from build123d import *

# Parameters (mm, degrees)
SKETCH1_W           = 166
SKETCH1_H           = 96
BOSS_EXTRUDE1_DEPTH = 18
SKETCH2_W           = 150
SKETCH2_H           = 80
CUT_EXTRUDE1_DEPTH  = 15
CUT_EXTRUDE5_DEPTH  = 10
FILLET1_R           = 4
FILLET2_R           = 4
FILLET5_R           = 1
CHAMFER1_SIZE       = 0.5


with BuildPart() as part:
    # Sketch1 → Boss-Extrude1 (new body)
    with BuildSketch(Plane(origin=(0, 0, 0), x_dir=(1, 0, 0), z_dir=(0, 1, 0))):
        with Locations((18.075570249, -18.706715624)):
            Rectangle(SKETCH1_W, SKETCH1_H)
    extrude(amount=BOSS_EXTRUDE1_DEPTH)

    # Sketch2 → Cut-Extrude1 (cut)
    with BuildSketch(Plane(origin=(0, 18, 0), x_dir=(1, 0, 0), z_dir=(0, 1, 0))):
        with Locations((18.075570249, -18.706715624)):
            Rectangle(SKETCH2_W, SKETCH2_H)
    extrude(amount=-CUT_EXTRUDE1_DEPTH, mode=Mode.SUBTRACT)

    # Sketch9 → Cut-Extrude5 (cut)
    with BuildSketch(Plane(origin=(0, 18, 0), x_dir=(1, 0, 0), z_dir=(0, 1, 0))):
        Polygon((-62.174429751, 26.543284376), (98.325570249, 26.543284376), (98.325570249, -58.706715624), (95.325570249, -58.706715624), (95.325570249, 23.543284376), (-59.174429751, 23.543284376), (-59.174429751, -58.706715624), (-62.174429751, -58.706715624), align=None)
    extrude(amount=-CUT_EXTRUDE5_DEPTH, mode=Mode.SUBTRACT)

    # Fillet1
    fillet1_edges = [part.edges().sort_by_distance(p)[0] for p in [
        (-64.924429751, 9, -29.293284376),
        (101.075570249, 9, -29.293284376),
        (101.075570249, 9, 66.706715624),
        (-64.924429751, 9, 66.706715624),
    ]]
    fillet(fillet1_edges, radius=FILLET1_R)

    # Fillet2
    fillet2_edges = [part.edges().sort_by_distance(p)[0] for p in [
        (-56.924429751, 10.5, 58.706715624),
        (-56.924429751, 10.5, -21.293284376),
        (93.075570249, 10.5, -21.293284376),
        (93.075570249, 10.5, 58.706715624),
    ]]
    fillet(fillet2_edges, radius=FILLET2_R)

    # Fillet5
    fillet5_edges = [part.edges().sort_by_distance(p)[0] for p in [
        (-64.924429751, 18, 18.706715624),
        (18.075570249, 18, -29.293284376),
        (18.075570249, 18, 66.706715624),
        (101.075570249, 18, 18.706715624),
        (-63.752856875, 18, 65.535142749),
        (99.903997374, 18, 65.535142749),
        (99.903997374, 18, -28.1217115),
        (-63.752856875, 18, -28.1217115),
        (93.075570249, 18, 18.706715624),
        (18.075570249, 18, 58.706715624),
        (18.075570249, 18, -21.293284376),
        (-56.924429751, 18, 18.706715624),
        (91.903997374, 18, 57.535142749),
        (91.903997374, 18, -20.1217115),
        (-55.752856875, 18, -20.1217115),
        (-55.752856875, 18, 57.535142749),
    ]]
    fillet(fillet5_edges, radius=FILLET5_R)

    # Chamfer1
    chamfer1_edges = [part.edges().sort_by_distance(p)[0] for p in [
        (-62.174429751, 18, 16.081715624),
        (-60.674429751, 18, 58.706715624),
        (-59.174429751, 18, 17.581715624),
        (18.075570249, 18, -23.543284376),
        (95.325570249, 18, 17.581715624),
        (96.825570249, 18, 58.706715624),
        (98.325570249, 18, 16.081715624),
        (18.075570249, 18, -26.543284376),
    ]]
    chamfer(chamfer1_edges, length=CHAMFER1_SIZE)


solid = part.part
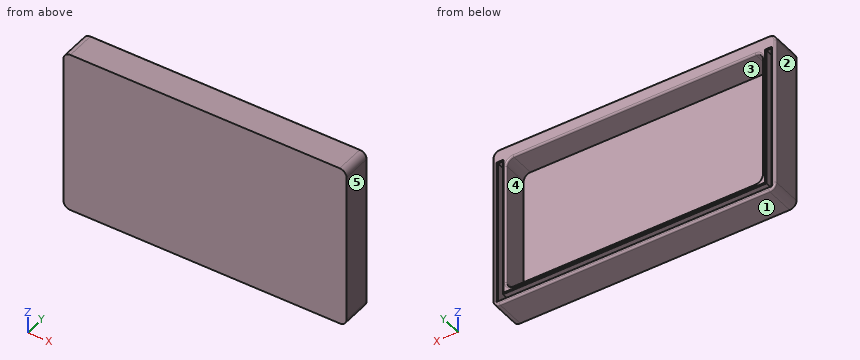
Read the model definition and answer for the solid it produces. Units are mm, in the model's axes. Face numbers are marked on the shaded views. A direction names the side the tool comes from. Coordinates: 2 decimals unless noted, no trailing zeros. Order: outer loops, then holes, each group sorted by start corner. A loop starts at its lowest first (then second) coordinate and runs counter-clockwise, first axis right, second up. Notation, with made-up numbers: (54.5, -11) -> (69.5, -11) arc R14 cw to (69.5, 0) -> close; hole circle Ø4 at (35, 47). An arc over 180 degrees is marked (long way). Answer as a JSON object with one key per item and string values.
1) A cutting plane is placed at D-D, the plane z = 49. Determine the outline of the cut face in (x, y).
Model answer:
{"outline": "(-64.92, 0) -> (101.08, 0) -> (101.08, 17) arc R1 ccw to (100.08, 18) -> (98.83, 18) -> (98.33, 17.5) -> (98.33, 8) -> (95.33, 8) -> (95.33, 17.5) -> (94.83, 18) -> (94.08, 18) arc R1 ccw to (93.08, 17) -> (93.08, 3) -> (-56.92, 3) -> (-56.92, 17) arc R1 ccw to (-57.92, 18) -> (-58.67, 18) -> (-59.17, 17.5) -> (-59.17, 8) -> (-62.17, 8) -> (-62.17, 17.5) -> (-62.67, 18) -> (-63.92, 18) arc R1 ccw to (-64.92, 17) -> close"}
2) The mould has two halves that part along Z. Classify the marked faces 1, 2 and 3: released by +Z, released by -Z, zero draft, split by the parting line, or undercut.
Model answer:
{"face 1": "released by -Z", "face 2": "zero draft", "face 3": "undercut"}
3) A tool of negligible diameter and unlimited length cuts with its end or side. For the marked faces 4 and 5, from which of +Z, -Z, +X, -X, +Y, -Y can it reach the whole face along a straight path? Write none if from no direction.
Model answer:
{"face 4": "+Y", "face 5": "+Z, -Z, +X, +Y, -Y"}
4) A cutting plane is placed at C-C, the plane y = 14.5. Determine the outline of the cut face in (x, z).
Model answer:
{"outline": "(-64.92, -25.29) arc R4 ccw to (-60.92, -29.29) -> (97.08, -29.29) arc R4 ccw to (101.08, -25.29) -> (101.08, 62.71) arc R4 ccw to (97.08, 66.71) -> (-60.92, 66.71) arc R4 ccw to (-64.92, 62.71) -> close; hole (-62.17, -26.54) -> (98.33, -26.54) -> (98.33, 58.71) -> (95.33, 58.71) -> (95.33, -23.54) -> (-59.17, -23.54) -> (-59.17, 58.71) -> (-62.17, 58.71) -> close; hole (-56.92, -17.29) arc R4 ccw to (-52.92, -21.29) -> (89.08, -21.29) arc R4 ccw to (93.08, -17.29) -> (93.08, 54.71) arc R4 ccw to (89.08, 58.71) -> (-52.92, 58.71) arc R4 ccw to (-56.92, 54.71) -> close"}
5) A cutting plane is placed at A-A, the plane y = 5.75. Determine the outline of the cut face in (x, z).
Model answer:
{"outline": "(-64.92, -25.29) arc R4 ccw to (-60.92, -29.29) -> (97.08, -29.29) arc R4 ccw to (101.08, -25.29) -> (101.08, 62.71) arc R4 ccw to (97.08, 66.71) -> (-60.92, 66.71) arc R4 ccw to (-64.92, 62.71) -> close; hole (-56.92, -17.29) arc R4 ccw to (-52.92, -21.29) -> (89.08, -21.29) arc R4 ccw to (93.08, -17.29) -> (93.08, 54.71) arc R4 ccw to (89.08, 58.71) -> (-52.92, 58.71) arc R4 ccw to (-56.92, 54.71) -> close"}
6) Each of these flat-tipped pins is pushed along its axis until it touches: pin 1 (1.5 mm diameter, centred on x = 41.5, z = 48, fed in from +Y); pin 2 (10 mm diameter, centred on x = -9.5, z = 11, fed in from -Y). Where does it stop, or does it pass through?
Model answer:
{"pin 1": "stops at y = 3", "pin 2": "stops at y = 0"}
7) Consider line 1 along Z through (x, y) = (0, 15); line 2 along X through (y, z) = (11.25, 2.5); line 3 along X through (y, z) = (6, -17). Determine where each line is inside the solid, lowest interval first. Write a range as from..to.
Model answer:
{"line 1": "z = -29.29..-26.54, -23.54..-21.29, 58.71..66.71", "line 2": "x = -64.92..-62.17, -59.17..-56.92, 93.08..95.33, 98.33..101.08", "line 3": "x = -64.92..-56.92, 93.08..101.08"}
8) A cutting plane is placed at B-B, the plane x = 61. Determine the outline of the cut face in (y, z), plus the area to 3 significant figures.
Model answer:
{"outline": "(0, -29.29) -> (17, -29.29) arc R1 ccw to (18, -28.29) -> (18, -27.04) -> (17.5, -26.54) -> (8, -26.54) -> (8, -23.54) -> (17.5, -23.54) -> (18, -23.04) -> (18, -22.29) arc R1 ccw to (17, -21.29) -> (3, -21.29) -> (3, 58.71) -> (17, 58.71) arc R1 ccw to (18, 59.71) -> (18, 65.71) arc R1 ccw to (17, 66.71) -> (0, 66.71) -> close", "area": "497 mm²"}
